Source: CAD feature listing. Evaluate the final solid. Frame: model axes, mm. A direction names the side the tool comes from. Round coordinates to 2 decimals unless told otherwise and drop trailing zeros. Loops run counter-clockwise (first coordinate to the right, second up) from the corner with the lowest first, then second, coordinate; pieces in that order, holes last. Notation, with made-up numbers: (-18, 17.25) -> (19, 17.25) arc R21 cw to (19, 28.25) -> close; hole circle Ø10 at (54, 66.25). An arc over 180 degrees is marked (long way). Put each result on its own line as item: value. Start each with the question number.
1. Cut plane B-B (y = 2.25). Return the cut outline in (x, z).
2. Cut plane A-A (x = -1.5). Return the cut outline in (y, z), then the cut area to 3 significant figures.
3. Contact query for flat-ended pins moving along their axis: pin 1 (6 mm diameter, centred on x = 6, y = -3.5, fed in from -Z); pin 2 (2 mm diameter, centred on x = -5, z = 2.5, fed in from -Y). Output: stop coordinate, or through.
4. Material intervals for L1, parallel to X at y = 0.25, z = 0.65; L2, parallel to Z at x = 0, y = 3.5; L3, parallel to X at y = 5, z = 0.6, sorted ascending.
5. Cut plane C-C (x = 1.75). Return the cut outline in (y, z), then the cut area to 3 significant figures.
6. Draft query along Y for faces 3 (the flat face through (-6.3, 5.2, 2)), 4 (the flat face through (6.3, -5.2, 1.7)), 5 (the flat face through (1, 0.6, 2)), 6 (the cylindrical face through (-2.548, 2.766, 1.983)). Return one class per face: pulls with the +Y half, pulls with the -Y half, needs draft (parallel to the pull), parting line crosses it, or undercut.
7. Set-up query: faces 1 (the cylindrical face through (3.89, -7.28, 1.58)), 2 (the flat face through (4.104, 3.153, 2.013)). Return all of +Z, -Z, +X, -X, +Y, -Y with unobstructed straight access to the full face (end or side cutting, diameter ignored); none if empty.
Autodesk Inventor part; units mm, degrees
ref_plane "YZ Plane" through (0, 0, 0) normal (1, 0, 0) x (0, 1, 0)
ref_plane "XZ Plane" through (0, 0, 0) normal (0, 1, 0) x (-1, 0, 0)
ref_plane "XY Plane" through (0, 0, 0) normal (0, 0, 1) x (1, 0, 0)
sketch "Base" plane through (0, 0, 0) normal (0, 0, 1) x (1, 0, 0)
  line L0 (-8.5, -3) -> (-8.5, 3)
  line L1 (-8.5, 3) -> (-4, 7.5)
  line L2 (-4, 7.5) -> (4, 7.5)
  line L3 (4, 7.5) -> (8.5, 3)
  line L4 (8.5, 3) -> (8.5, -3)
  line L5 (8.5, -3) -> (4, -7.5)
  line L6 (4, -7.5) -> (-4, -7.5)
  line L7 (-4, -7.5) -> (-8.5, -3)
  line L8 (-8.5, 0) -> (8.5, 0) construction
  line L9 (0, 7.5) -> (0, -7.5) construction
  point P0 (0, 0)
  point P1 (0, 0)
  dimension "d1" = 17
  dimension "d5" = 15
  dimension "d7" = 6
extrude "BaseFeature" add sketch "Base" along normal blind 4
fillet "BaseFilletsFeature" radius 3 8 edges at (-8.5, -3, 2) (-4, -7.5, 2) (4, -7.5, 2) (8.5, -3, 2) (8.5, 3, 2) (4, 7.5, 2) (-4, 7.5, 2) (-8.5, 3, 2)
sketch "RailHoles" plane through (0, 0, 4) normal (0, 0, 1) x (1, 0, 0)
  line L0 (1.6663, 4.1769) -> (5.1769, 0.6663) construction
  line L1 (-1.8568, 2.0431) -> (1.6538, -1.4675) construction
  line L2 (7.6213, 3.8787) -> (4.8787, 6.6213) construction
  line L3 (6.25, 5.25) -> (3.4216, 2.4216) construction
  circle A0 centre (1.6663, 4.1769) radius 1
  circle A1 centre (5.1769, 0.6663) radius 1
  circle A2 centre (-1.8568, 2.0431) radius 1
  circle A3 centre (1.6538, -1.4675) radius 1
  line L4 (2.3734, 4.884) -> (5.884, 1.3734)
  line L5 (0.9592, 3.4698) -> (4.4698, -0.0408)
  line L6 (-1.1497, 2.7502) -> (2.3609, -0.7604)
  line L7 (-2.5639, 1.336) -> (0.9467, -2.1746)
  dimension "d11" = 4
  dimension "d12" = 4
  dimension "d13" = 4.9647
  dimension "d14" = 2
  dimension "d15" = 1.5
  dimension "d25" = 3.8787
extrude "RailHolesFeature" cut sketch "RailHoles" against normal through all
sketch "RouteHole" plane through (-2.7574, -7.5, 0) normal (0, -1, 0) x (1, 0, 0)
  line L0 (5.5147, 4) -> (5.5147, 0) construction
  line L1 (0, 4) -> (5.5147, 4) construction
  line L2 (0, 0) -> (0, 4) construction
  line L3 (5.5147, 0) -> (0, 0) construction
  line L4 (0, 4) -> (0, 0) construction
  line L5 (0, 4) -> (5.5147, 4) construction
  line L6 (2.7574, 4) -> (2.7574, 0) construction
  line L7 (5.5147, 0) -> (0, 0) construction
  circle A0 centre (2.7574, 1.5) radius 1.25
  dimension "d40" = 2.5
  dimension "d41" = 1.5
hole "RouteHoleFeature" at (0, -7.5, 1.5) direction (0, 1, 0) diameter 2 end through all
sketch "SideProfile" plane through (8.5, -1.7574, 0) normal (1, 0, 0) x (0, 0, -1)
  arc A0 (-4, 9.2574) -> (-3, -5.7426) centre (109, 9.2574) ccw
  line L0 (-4, -5.7426) -> (0, -5.7426) construction
  line L1 (0, 9.2574) -> (-4, 9.2574) construction
  line L2 (-3, -5.7426) -> (0, -5.7426)
  line L3 (0, 9.2574) -> (0, -5.7426)
  line L4 (0, 9.2574) -> (0, 8.3787)
  line L5 (0, 9.2574) -> (-4, 9.2574)
  line L6 (-4, -2.1213) -> (-4, 0) construction
  dimension "d36" = 4
  dimension "d39" = 3
extrude "SideProfileFeature" cut sketch "SideProfile" against normal through all keep common part
equation "\"d7\" = 0.4 * d5"
equation "\"d12\" = 2 * d14"
equation "\"d13\" = 1.28 * d25"
properties part number "MiddleRouter"
Solution:
1. outline: (-8.46, 0) -> (-2.84, 0) -> (-2.84, 3.88) -> (-8.46, 3.88) -> close; (-0.65, 0) -> (2.18, 0) -> (2.18, 3.88) -> (-0.65, 3.88) -> (-0.65, 2.26) arc R1 cw (long way) to (-0.65, 0.74) -> close; (5.01, 0) -> (8.46, 0) -> (8.46, 3.88) -> (5.01, 3.88) -> close
2. outline: (-7.5, 0) -> (0.27, 0) -> (0.27, 3.77) arc R113 ccw to (-7.5, 3) -> close; (2.98, 0) -> (7.5, 0) -> (7.5, 4) arc R113 ccw to (2.98, 3.91) -> close
2. area: 44.6 mm^2
3. pin 1: stops at z = 0
3. pin 2: stops at y = -7.23
4. L1: x = -8.5 to -1.48, 1.35 to 4.18, 6.09 to 8.5
4. L2: z = 0 to 0.5, 2.5 to 3.93
4. L3: x = -6.5 to -0.44, 0.44 to 1.1, 2.23 to 6.5
5. outline: (-7.5, 0) -> (-2.46, 0) -> (-2.46, 3.56) arc R113 ccw to (-7.5, 3) -> close; (-0.15, 0) -> (2.68, 0) -> (2.68, 3.9) arc R113 ccw to (-0.15, 3.74) -> close; (5.17, 0) -> (7.5, 0) -> (7.5, 4) arc R113 ccw to (5.17, 3.98) -> close
5. area: 36.7 mm^2
6. face 3: pulls with the +Y half
6. face 4: pulls with the -Y half
6. face 5: undercut
6. face 6: undercut
7. face 1: +Z, -Z, +X, -Y
7. face 2: +Z, -Z
